Here's how the part is built. I have some questions about the finished solid (model axes, mm). A direction names the side the tool comes from. Give positions to 0.01 mm unless a question says otherwise; leave off trailing zeros. Order: outer loops, then holes, each group sorted by start corner. A loop starts at its lowest first (then second) coordinate and runs counter-clockwise, first axis right, second up. Notation, with made-up numbers: M 27,59 L 41,59 A12 ccw 41,75 Z; hole C 59.5,-22 d3. An arc over 180 degrees is marked long. Use one line per item in the form item = value.
Autodesk Inventor part; units mm, degrees
ref_plane "YZ Plane" through (0, 0, 0) normal (1, 0, 0) x (0, 1, 0)
ref_plane "XZ Plane" through (0, 0, 0) normal (0, 1, 0) x (-1, 0, 0)
ref_plane "XY Plane" through (0, 0, 0) normal (0, 0, 1) x (1, 0, 0)
sketch "Sketch1" plane through (0, 0, 0) normal (0, 1, 0) x (-1, 0, 0)
  point P0 (0, 0)
sketch "Sketch6" plane through (0, 0, 0) normal (0, 0, 1) x (1, 0, 0)
  line L0 (0, 0) -> (184, 0)
  line L1 (184, 0) -> (184, 61.2)
  line L2 (184, 61.2) -> (0, 61.2)
  line L3 (0, 61.2) -> (0, 0)
  line L4 (0, 0) -> (184, 0)
  line L5 (184, 0) -> (184, 61.2)
  dimension "d18" = 184
  dimension "d19" = 61.2
extrude "Extrusion5" add sketch "Sketch6" along normal blind 2
sketch "Sketch7" plane through (0, 0, 2) normal (0, 0, 1) x (1, 0, 0)
  line L0 (184, 61.2) -> (0, 61.2)
  line L1 (0, 61.2) -> (0, 30.6)
  line L2 (0, 30.6) -> (2.5, 30.6)
  line L3 (2.5, 30.6) -> (2.5, 38.1)
  line L4 (2.5, 30.6) -> (2.5, 23.1)
  line L5 (2.5, 38.1) -> (7.5, 38.1)
  line L6 (7.5, 38.1) -> (7.5, 23.1)
  line L7 (7.5, 23.1) -> (2.5, 23.1)
  point P0 (0, 0)
  dimension "d22" = 30.6
  dimension "d23" = 2.5
  dimension "d24" = 7.5
  dimension "d25" = 7.5
  dimension "d26" = 5
extrude "Extrusion6" add sketch "Sketch7" along normal blind 7
sketch "Sketch8" plane through (0, 0, 2) normal (0, 0, 1) x (1, 0, 0)
  line L0 (184, 61.2) -> (0, 61.2)
  line L1 (184, 61.2) -> (191, 61.2)
  line L2 (191, 61.2) -> (191, 0)
  line L3 (191, 0) -> (184, 0)
  line L4 (184, 0) -> (184, 61.2)
  point P0 (0, 0)
  dimension "d29" = 7
extrude "Extrusion7" add sketch "Sketch8" against normal blind 2
sketch "Sketch2" plane through (0, 0, 0) normal (0, 1, 0) x (-1, 0, 0)
  line L0 (0, 0) -> (92.58, 0)
  line L1 (92.58, 0) -> (92.58, -29.35)
  line L2 (92.58, -29.35) -> (0, -29.35)
  line L3 (0, -29.35) -> (0, 29.35)
  line L4 (0, 29.35) -> (92.58, 29.35)
  line L5 (92.58, 29.35) -> (92.58, -29.35)
  dimension "d0" = 92.58
  dimension "d1" = 29.35
  dimension "d2" = 92.58
  dimension "d3" = 58.7
sketch "Sketch3" plane through (0, 3, 0) normal (0, 1, 0) x (1, 0, 0)
  line L0 (0, 0) -> (-10, 0)
  line L1 (-10, 0) -> (-10, 7.5)
  line L2 (-10, 7.5) -> (-15, 7.5)
  line L3 (-15, 7.5) -> (-15, -7.5)
  line L4 (-15, -7.5) -> (-10, -7.5)
  line L5 (-10, -7.5) -> (-10, 7.5)
  dimension "d6" = 10
  dimension "d7" = 7.5
  dimension "d8" = 5
  dimension "d9" = 15
sketch "Sketch4" plane through (0, 3, 0) normal (0, 1, 0) x (1, 0, 0)
  line L0 (0, -29.35) -> (0, 29.35)
  line L1 (0, -29.35) -> (0, -34.35)
  line L2 (0, -34.35) -> (-5, -34.35)
  line L3 (-5, -34.35) -> (-5, -29.35)
  line L4 (-92.58, -29.35) -> (0, -29.35)
  line L5 (-5, -29.35) -> (0, -29.35)
  point P0 (0, 0)
  dimension "d12" = 5
  dimension "d13" = 5
sketch "Sketch5" plane through (0, 8, 0) normal (0, 1, 0) x (1, 0, 0)
  line L0 (-15, 7.5) -> (-15, -7.5)
  line L1 (-10, -7.5) -> (-10, 7.5)
  line L2 (-15, 7.5) -> (-10, 7.5)
  line L3 (-10, 7.5) -> (-10, -7.5)
  line L4 (-10, -7.5) -> (-15, -7.5)
  line L5 (-15, -7.5) -> (-15, 7.5)
  point P0 (0, 0)
equation "\"d2\" = d0"
equation "\"d3\" = 2 * d1"
equation "\"d9\" = 2 * d7"
properties part number "Door"
Q1. I want a section at B-B on x = 47. Write out the boundary of the cut face in (y, z), then the cut area to 3 significant figures.
Found:
outline = M 0,0 L 61.2,0 L 61.2,2 L 0,2 Z
area = 122 mm²
Q2. I want a section at A-A on y = 35. Write out the boundary of the cut face in (x, z), then the cut area to 3 significant figures.
Found:
outline = M 0,0 L 191,0 L 191,2 L 7.5,2 L 7.5,9 L 2.5,9 L 2.5,2 L 0,2 Z
area = 417 mm²
Q3. I want a section at C-C on z = 3.5. Write out the boundary of the cut face in (x, y).
Found:
outline = M 2.5,23.1 L 7.5,23.1 L 7.5,38.1 L 2.5,38.1 Z
Q4. On a 3-axis mill with a long thin cutter (end or side, diameter ignored), from which of +Z, -Z, +X, -X, +Y, -Y can I reach the whole of each face in a straight line? I mean faces 1 (the face through (2.5, 31, 5)), 2 (the face through (5, 38.1, 5)), 3 (the face through (7.5, 31, 5)), 4 (the face through (5, 23.1, 5)). Say none if no direction works.
Found:
face_1 = +Z, -X, +Y, -Y
face_2 = +Z, +X, -X, +Y
face_3 = +Z, +X, +Y, -Y
face_4 = +Z, +X, -X, -Y
Q5. I need wall thicknesses on L1, parallel to X at y = 27, z = 5.75; L2, parallel to Z at x = 140, y = 21.5. Which ranges of each line are inside material? Lowest first, please.
Found:
L1 = 2.5 to 7.5
L2 = 0 to 2
Q6. I'm going to push flat-ended pins straight in: pin 1 Ø5 at (x, y) = (171.5, 24) entering from -Z; pin 2 Ø18.5 at (x, y) = (93, 39.5) entering from +Z; pin 3 Ø1 at (y, z) = (33.5, 3.5) entering from +X; pin 4 Ø2.5 at (x, z) = (5.5, 4) entering from -Y. Where does each tip first touch, or does it pass through?
Found:
pin_1 = 0
pin_2 = 2
pin_3 = 7.5
pin_4 = 23.1
